```python
from build123d import *

# Parameters (mm, degrees)
BOSS_EXTRUDE1_DEPTH                                 = 2
FILLET1_R                                           = 2.5
SKETCH2_W                                           = 8
SKETCH2_H                                           = 15
CUT_EXTRUDE1_DEPTH                                  = 2
CUT_EXTRUDE2_DEPTH                                  = 1
FILLET3_SIZE                                        = 0.5
FILLET4_SIZE                                        = 0.5
CUT_EXTRUDE3_DEPTH                                  = 50.157908825
FILLET5_SIZE                                        = 0.5
CSK_FOR_M2_COUNTERSUNK_FLAT_HEAD_SCREW1_D           = 2.4
CSK_FOR_M2_COUNTERSUNK_FLAT_HEAD_SCREW1_DEPTH       = 4.278967257
CSK_FOR_M2_COUNTERSUNK_FLAT_HEAD_SCREW1_CSINK_D     = 4.4
CSK_FOR_M2_COUNTERSUNK_FLAT_HEAD_SCREW1_CSINK_ANGLE = 90
CSK_FOR_M2_COUNTERSUNK_FLAT_HEAD_SCREW1_TIP         = 0.721032743
CSK_FOR_M2_COUNTERSUNK_FLAT_HEAD_SCREW2_D           = 2.4
CSK_FOR_M2_COUNTERSUNK_FLAT_HEAD_SCREW2_DEPTH       = 4.278967257
CSK_FOR_M2_COUNTERSUNK_FLAT_HEAD_SCREW2_CSINK_D     = 4.4
CSK_FOR_M2_COUNTERSUNK_FLAT_HEAD_SCREW2_CSINK_ANGLE = 90
CSK_FOR_M2_COUNTERSUNK_FLAT_HEAD_SCREW2_TIP         = 0.721032743


with BuildPart() as part:
    # Sketch1 → Boss-Extrude1 (new body)
    with BuildSketch(Plane(origin=(0, 0, 0), x_dir=(1, 0, 0), z_dir=(0, 1, 0))):
        Polygon((-47.5, 6.5), (-41.5, 12.5), (41.5, 12.5), (47.5, 6.5), (47.5, -6.5), (41.5, -12.5), (-41.5, -12.5), (-47.5, -6.5), align=None)
    extrude(amount=BOSS_EXTRUDE1_DEPTH)

    # Fillet1
    fillet1_edges = [part.edges().sort_by_distance(p)[0] for p in [
        (41.5, 1, -12.5),
        (47.5, 1, -6.5),
        (47.5, 1, 6.5),
        (41.5, 1, 12.5),
        (-41.5, 1, 12.5),
        (-47.5, 1, 6.5),
        (-47.5, 1, -6.5),
        (-41.5, 1, -12.5),
    ]]
    fillet(fillet1_edges, radius=FILLET1_R)

    # Sketch2 → Cut-Extrude1 (cut)
    with BuildSketch(Plane(origin=(0, 2, 0), x_dir=(1, 0, 0), z_dir=(0, 1, 0))):
        Rectangle(SKETCH2_W, SKETCH2_H)
    extrude(amount=-CUT_EXTRUDE1_DEPTH, mode=Mode.SUBTRACT)

    # Sketch3 → Cut-Extrude2 (cut)
    with BuildSketch(Plane(origin=(0, 2, 0), x_dir=(1, 0, 0), z_dir=(0, 1, 0))):
        with BuildLine():
            Line((-5, -10), (5, -10))
            ThreePointArc((5, -10), (8.535533906, -8.535533906), (10, -5))
            Line((10, -5), (10, 5))
            ThreePointArc((10, 5), (8.535533906, 8.535533906), (5, 10))
            Line((5, 10), (-5, 10))
            ThreePointArc((-5, 10), (-8.535533906, 8.535533906), (-10, 5))
            Line((-10, 5), (-10, -5))
            ThreePointArc((-10, -5), (-8.535533906, -8.535533906), (-5, -10))
        make_face()
    extrude(amount=-CUT_EXTRUDE2_DEPTH, mode=Mode.SUBTRACT)

    # Fillet3
    fillet3_edges = [part.edges().sort_by_distance(p)[0] for p in [
        (-8.535533906, 1, 8.535533906),
        (-10, 1, 0),
        (-8.535533906, 1, -8.535533906),
        (0, 1, -10),
        (8.535533906, 1, -8.535533906),
        (10, 1, 0),
        (8.535533906, 1, 8.535533906),
        (0, 1, 10),
    ]]
    chamfer(fillet3_edges, length=FILLET3_SIZE)

    # Fillet4
    fillet4_edges = [part.edges().sort_by_distance(p)[0] for p in [
        (0, 2, 12.5),
        (-44.5, 2, 9.5),
        (0, 2, -12.5),
        (-44.5, 2, -9.5),
        (-47.5, 2, 0),
        (44.5, 2, 9.5),
        (47.5, 2, 0),
        (44.5, 2, -9.5),
        (41.421174675, 2, 12.309698831),
        (47.309698831, 2, 6.421174675),
        (47.309698831, 2, -6.421174675),
        (41.421174675, 2, -12.309698831),
        (-41.421174675, 2, -12.309698831),
        (-47.309698831, 2, -6.421174675),
        (-47.309698831, 2, 6.421174675),
        (-41.421174675, 2, 12.309698831),
    ]]
    chamfer(fillet4_edges, length=FILLET4_SIZE)

    # Sketch5 → Cut-Extrude3 (cut, through all)
    with BuildSketch(Plane(origin=(0, 2, 0), x_dir=(1, 0, 0), z_dir=(0, 1, 0))):
        with BuildLine():
            Line((39.98959236, 9.060660172), (37.868272016, 6.939339828))
            ThreePointArc((37.868272016, 6.939339828), (37.575378798, 6.232233047), (37.868272016, 5.525126266))
            Line((37.868272016, 5.525126266), (41.454058454, 1.939339828))
            ThreePointArc((41.454058454, 1.939339828), (42.161165235, 1.646446609), (42.868272016, 1.939339828))
            Line((42.868272016, 1.939339828), (44.98959236, 4.060660172))
            ThreePointArc((44.98959236, 4.060660172), (45.282485579, 4.767766953), (44.98959236, 5.474873734))
            Line((44.98959236, 5.474873734), (41.403805922, 9.060660172))
            ThreePointArc((41.403805922, 9.060660172), (40.696699141, 9.353553391), (39.98959236, 9.060660172))
        make_face()
    extrude(amount=-CUT_EXTRUDE3_DEPTH, mode=Mode.SUBTRACT)

    # Fillet5
    fillet5_edges = [part.edges().sort_by_distance(p)[0] for p in [
        (40.696699141, 2, -9.353553391),
        (43.196699141, 2, -7.267766953),
        (45.282485579, 2, -4.767766953),
        (43.928932188, 2, -3),
        (42.161165235, 2, -1.646446609),
        (38.928932188, 2, -8),
        (37.575378798, 2, -6.232233047),
        (39.661165235, 2, -3.732233047),
    ]]
    chamfer(fillet5_edges, length=FILLET5_SIZE)

    # CSK for M2 Countersunk Flat Head Screw1
    with Locations(Plane(origin=(36.5, 2, 0), x_dir=(0, 0, 1), z_dir=(0, 1, 0))):
        with Locations((0, 0)):
            CounterSinkHole(CSK_FOR_M2_COUNTERSUNK_FLAT_HEAD_SCREW1_D / 2, CSK_FOR_M2_COUNTERSUNK_FLAT_HEAD_SCREW1_CSINK_D / 2, depth=CSK_FOR_M2_COUNTERSUNK_FLAT_HEAD_SCREW1_DEPTH, counter_sink_angle=CSK_FOR_M2_COUNTERSUNK_FLAT_HEAD_SCREW1_CSINK_ANGLE)
            with Locations((0, 0, -(CSK_FOR_M2_COUNTERSUNK_FLAT_HEAD_SCREW1_DEPTH + CSK_FOR_M2_COUNTERSUNK_FLAT_HEAD_SCREW1_TIP / 2))):  # 118° drill point
                Cone(0, CSK_FOR_M2_COUNTERSUNK_FLAT_HEAD_SCREW1_D / 2, CSK_FOR_M2_COUNTERSUNK_FLAT_HEAD_SCREW1_TIP, mode=Mode.SUBTRACT)

    # CSK for M2 Countersunk Flat Head Screw2
    with Locations(Plane(origin=(-36.5, 2, -6.5), x_dir=(0, 0, 1), z_dir=(0, 1, 0))):
        with Locations((0, 0), (13, 0)):
            CounterSinkHole(CSK_FOR_M2_COUNTERSUNK_FLAT_HEAD_SCREW2_D / 2, CSK_FOR_M2_COUNTERSUNK_FLAT_HEAD_SCREW2_CSINK_D / 2, depth=CSK_FOR_M2_COUNTERSUNK_FLAT_HEAD_SCREW2_DEPTH, counter_sink_angle=CSK_FOR_M2_COUNTERSUNK_FLAT_HEAD_SCREW2_CSINK_ANGLE)
            with Locations((0, 0, -(CSK_FOR_M2_COUNTERSUNK_FLAT_HEAD_SCREW2_DEPTH + CSK_FOR_M2_COUNTERSUNK_FLAT_HEAD_SCREW2_TIP / 2))):  # 118° drill point
                Cone(0, CSK_FOR_M2_COUNTERSUNK_FLAT_HEAD_SCREW2_D / 2, CSK_FOR_M2_COUNTERSUNK_FLAT_HEAD_SCREW2_TIP, mode=Mode.SUBTRACT)


solid = part.part
```
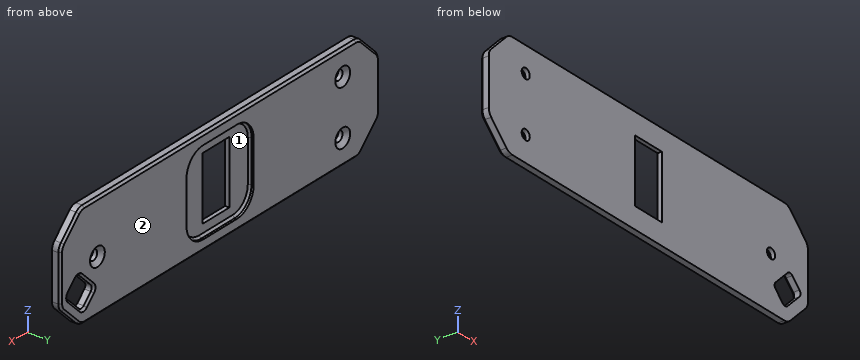
Work out the finished part from the listing and answer in its coordinate system (mm). Face numbers are marked on the shaded views. Round coordinates to 2 decimals unless told otherwise and drop trailing zeros. Loops run counter-clockwise (first coordinate to the right, second up) from the corner with the lowest first, then second, coordinate; pieces in that order, holes last.
(1) Each of these flat-tipped pins is pushed along its axis until it touches: P1, Ø2, axis at x = -36.5, z = 6.5, coming from the -Y side; P2, Ø3, axis at x = -36.5, z = -6.5, coming from the +Y side; P3, Ø3, axis at x = 6.5, z = 0, coming from the +Y side; P4, Ø0.6, axis at x = 2, y = 2, coming from the +Z side. Where does it stop, or does it pass through?
Computed values:
P1: passes through
P2: stops at y = 1.3
P3: stops at y = 1
P4: stops at z = 12.3
(2) The part is cut by section A-A, the plane z = 0. Give the vertices of the cut face in (x, y).
Computed values:
outline: (-47.5, 0) - (-4, 0) - (-4, 1) - (-9.5, 1) - (-10, 1.5) - (-10, 2) - (-47, 2) - (-47.5, 1.5) - close; (4, 0) - (35.3, 0) - (35.3, 1) - (34.3, 2) - (10, 2) - (10, 1.5) - (9.5, 1) - (4, 1) - close; (37.7, 0) - (47.5, 0) - (47.5, 1.5) - (47, 2) - (38.7, 2) - (37.7, 1) - close
(3) The part is cut by section B-B, the plane x = -36.5. Give the vertices of the cut face in (y, z), and give its area (4 significant figures).
Computed values:
outline: (0, -12.5) - (1.5, -12.5) - (2, -12) - (2, -8.7) - (1, -7.7) - (0, -7.7) - close; (0, -5.3) - (1, -5.3) - (2, -4.3) - (2, 4.3) - (1, 5.3) - (0, 5.3) - close; (0, 7.7) - (1, 7.7) - (2, 8.7) - (2, 12) - (1.5, 12.5) - (0, 12.5) - close
area: 38.15 mm2
(4) Find the intervals of material crossed by L1, parallel to Z at x = -36.5, y = 0.3; L2, parallel to X at y = 0.25, z = 0; L3, parallel to X at y = 0.3, z = -1.75, in increasing order.
Computed values:
L1: z = -12.5 to -7.7, -5.3 to 5.3, 7.7 to 12.5
L2: x = -47.5 to -4, 4 to 35.3, 37.7 to 47.5
L3: x = -47.5 to -4, 4 to 41.72, 42.6 to 47.5
(5) The mould has two halves that part along X. Classify the marked faces 1 and 2: pulls with the +X half, pulls with the -X half, needs draft (parallel to the pull), parting line crosses it, or undercut.
Computed values:
face 1: undercut
face 2: needs draft
